Geometry: final body of the model. Coordinates: model frame, mm. A direction names the side the tool comes from. Give positions to 0.01 mm unless a question says otherwise; leave off trailing zeros. Loops run counter-clockwise (first coordinate to the right, second up) from the corner with the lowest first, then second, coordinate; pieces in that order, holes last. Notation, with made-up numbers: (26.5, -37) -> (41.5, -37) arc R21 cw to (41.5, -33) -> close; hole circle Ø2 at (87, 5). An arc over 180 degrees is marked (long way). Answer in a Markdown table with one row per item. Add a question column.
1) Line query: line 1 (X direction, y = 11.75, z = 7.5); line 2 (X direction, y = 7, z = 5); line 3 (Y direction, x = 5, z = 8.75). Output: solid intervals per line, ascending. Write a range as from..to.
2) Section query B-B (z = 1). Return the cut outline in (x, y).
3) Section query D-D (x = 5). Return the cut outline in (y, z), plus the area to 3 significant figures.
4) Section query A-A (y = 8.75). Return the cut outline in (x, z), plus the area to 3 significant figures.
5) Access query for faces 1 (the flat face through (9, 12, 6)), 2 (the flat face through (7, 10, 6)). Directions: +Z, -Z, +X, -X, +Y, -Y. A direction counts if a zero-diameter tool reaches every point of the face in a straight line with its end or side. Return the directions, or none.
6) Section query C-C (y = 7). Return the cut outline in (x, z).
7) Draft query along Y for faces 3 (the flat face through (2, 12, 6)), 4 (the flat face through (5, 3, 0)), 5 (the cylindrical face through (5.1, 4.5, 5.9)), 6 (the flat face through (5, 0, 6)). Return one class per face: +Y half, -Y half, draft (parallel to the pull), parting line (faces both ways), or undercut.
Autodesk Fusion 360 part; units mm, degrees
sketch "Sketch1" plane through (0, 0, 0) normal (0, 0, 1) x (1, 0, 0)
  line L0 (0, 0) -> (10, 0)
  line L1 (10, 0) -> (10, 12)
  line L2 (10, 12) -> (0, 12)
  line L3 (0, 12) -> (0, 0)
  line L4 (5, 0) -> (5, 7)
  circle A0 centre (5, 7) radius 2.5
  line L5 (5, 7) -> (7, 7)
  line L6 (7, 7) -> (7, 12)
  line L7 (3, 7) -> (3, 12)
  dimension "d1" = 10
  dimension "d2" = 12
  dimension "d3" = 7
  dimension "d4" = 5
  dimension "d5" = 2
extrude "Extrude1" add sketch "Sketch1" along normal blind 12 contours L0 L2 L3 L4 A0 L7 | L0 L1 L2 L4 A0 L6
Evaluation:
| question | item | result |
|---|---|---|
| 1 | line 1 | 0..3, 7..10 |
| 1 | line 2 | 0..2.5, 7.5..10 |
| 1 | line 3 | 0..4.5 |
| 2 | outline | (0, 0) -> (10, 0) -> (10, 12) -> (7, 12) -> (7, 8.5) arc R2.5 cw (long way) to (3, 8.5) -> (3, 12) -> (0, 12) -> close |
| 3 | outline | (0, 0) -> (4.5, 0) -> (4.5, 12) -> (0, 12) -> close |
| 3 | area | 54.0 mm² |
| 4 | outline | (0, 0) -> (3, 0) -> (3, 12) -> (0, 12) -> close; (7, 0) -> (10, 0) -> (10, 12) -> (7, 12) -> close |
| 4 | area | 72.0 mm² |
| 5 | face 1 | +Z, -Z, +X, -X, +Y |
| 5 | face 2 | +Z, -Z, +Y |
| 6 | outline | (0, 0) -> (2.5, 0) -> (2.5, 12) -> (0, 12) -> close; (7.5, 0) -> (10, 0) -> (10, 12) -> (7.5, 12) -> close |
| 7 | face 3 | +Y half |
| 7 | face 4 | draft |
| 7 | face 5 | undercut |
| 7 | face 6 | -Y half |
